Work out the finished part from the listing and answer in its coordinate system (mm). Face numbers are marked on the shaded views. A direction names the side the tool comes from. Give positions to 0.01 mm unless a question says otherwise; leave off trailing zeros. Loops run counter-clockwise (first coordinate to the right, second up) from the corner with the lowest first, then second, coordinate; pieces in that order, holes last.
from build123d import *

# Parameters (mm, degrees)
F0_W          = 456
F0_H          = 456
F0_W_2        = 450
F0_H_2        = 450
F2_DEPTH      = 1000
F3_DEPTH      = 228.001
F3_DEPTH_BACK = 228.001
F5_DEPTH      = 456.001


with BuildPart() as f2:
    # F0 (on Top) → F2 (new body)
    with BuildSketch(Plane.XY):
        Rectangle(F0_W, F0_H)
        Rectangle(F0_W_2, F0_H_2, mode=Mode.SUBTRACT)
    extrude(amount=F2_DEPTH)

    # F1 (on Right) → F3 (cut, two sides)
    with BuildSketch(Plane.YZ) as f3_sk:
        Polygon((-228, -173.997311), (228, -173.997311), (228, 186.002689), (-228, 0), align=None)
    extrude(amount=F3_DEPTH, mode=Mode.SUBTRACT)
    extrude(f3_sk.sketch, amount=-F3_DEPTH_BACK, mode=Mode.SUBTRACT)

    # F4 (on face) → F5 (cut, through all)
    with BuildSketch(Plane.YZ.offset(228)):
        Polygon((-228, 1000), (-228, 820), (228, 1000), align=None)
    extrude(amount=-F5_DEPTH, mode=Mode.SUBTRACT)


solid = f2.part
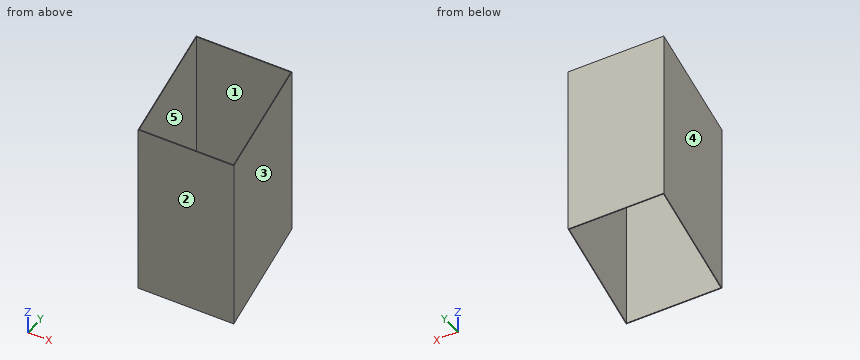
Item 1: For the marked faces 1 and 2, determine the directions among +Z, -Z, +X, -X, +Y, -Y from which every point of the face is accessible in a straight line to the end or side of a thin tool.
Item 2: Determine the mould class of the marked faces 3, 4 and 5 for opening direction X: released by +X, released by -X, zero draft, split by the parting line, or undercut.
Item 3: Find section A-A, the plane x = 199. Write down the section's boundary in (y, z), plus the area to 3 significant figures.
Item 4: Find section D-D, the plane z = 169. Write down the section's boundary in (x, y).
Item 5: Find section B-B, the plane z = 538. Write down the section's boundary in (x, y), plus the area to 3 significant figures.
Item 6: Consider line 1 (Y direction, x = -28, z = 205); line 2 (Y direction, x = 127.5, z = 51). Determine where each line is inside the solid, lowest interval first.
Item 7: Find section C-C, the plane y = -44. Write down the section's boundary in (x, z).
Ans:
1. face 1: +Z, -Z
1. face 2: +Z, -Z, +X, -X, -Y
2. face 3: released by +X
2. face 4: released by -X
2. face 5: undercut
3. outline: (-228, 0) - (-225, 1.22) - (-225, 821.18) - (-228, 820) - close; (225, 184.78) - (228, 186) - (228, 1000) - (225, 998.82) - close
3. area: 4,900 mm2
4. outline: (-228, -228) - (228, -228) - (228, 186.32) - (225, 186.32) - (225, -225) - (-225, -225) - (-225, 186.32) - (-228, 186.32) - close
5. outline: (-228, -228) - (228, -228) - (228, 228) - (-228, 228) - close; hole (-225, -225) - (225, -225) - (225, 225) - (-225, 225) - close
5. area: 5,440 mm2
6. line 1: y = -228 to -225, 225 to 228
6. line 2: y = -228 to -225
7. outline: (-228, 75.05) - (-225, 75.05) - (-225, 892.63) - (-228, 892.63) - close; (225, 75.05) - (228, 75.05) - (228, 892.63) - (225, 892.63) - close
